Build history of the part. All positions in model axes, mm. A direction names the side the tool comes from. Coordinates: 2 decimals unless noted, no trailing zeros. Order: outer loops, then holes, each group sorted by start corner. A loop starts at its lowest first (then second) coordinate and runs counter-clockwise, first axis right, second up. Notation, with made-up numbers: (35, -18.5) - (77, -18.5) arc R18 ccw to (77, 12.5) - close; hole circle Ø4 at (-17, 80.25). An arc over 180 degrees is marked (long way). One line per item, written item: value.
Autodesk Inventor part; units mm, degrees
ref_plane "YZ Plane" through (0, 0, 0) normal (1, 0, 0) x (0, 1, 0)
ref_plane "XZ Plane" through (0, 0, 0) normal (0, 1, 0) x (-1, 0, 0)
ref_plane "XY Plane" through (0, 0, 0) normal (0, 0, 1) x (1, 0, 0)
sketch "草圖1" plane through (0, 0, 0) normal (0, 0, 1) x (1, 0, 0)
  circle A0 centre (0, 0) radius 20
  line L0 (0, -20) -> (0, -30)
  line L1 (0, -30) -> (70, -30)
  line L2 (70, -30) -> (70, -20)
  line L3 (70, -20) -> (40, 20)
  line L4 (40, 20) -> (0, 20)
  dimension "d0" = 40
  dimension "d1" = 10
  dimension "d2" = 70
  dimension "d3" = 40
  dimension "d4" = 10
extrude "擠出1" add sketch "草圖1" along normal blind 10
sketch "草圖2" plane through (0, 0, 10) normal (0, 0, 1) x (1, 0, 0)
  arc A0 (0, 20) -> (0, -20) centre (0, 0) ccw
hole "孔1" at (0, 0, 10) direction (0, 0, -1) diameter 20 end through all
sketch "草圖3" plane through (0, -30, 0) normal (0, -1, 0) x (1, 0, 0)
  line L0 (70, 10) -> (70, 0)
  line L1 (70, 0) -> (0, 0)
  line L2 (0, 0) -> (0, 10)
  line L3 (0, 10) -> (70, 10)
  circle A0 centre (20, 30) radius 20
  line L4 (0, 30) -> (40, 30)
  line L5 (40, 30) -> (40, 0)
  line L6 (40, 0) -> (0, 0)
  line L7 (0, 0) -> (0, 30)
  line L8 (0, 0) -> (70, 0)
  line L9 (0, 0) -> (0, 10)
  point P0 (40, 10)
  point P1 (40, 30)
  dimension "d14" = 40
  dimension "d15" = 30
extrude "擠出2" add sketch "草圖3" against normal blind 10 contours L3 A0 L5 | L3 L7 A0 | A0 L4 | L4 A0
sketch "草圖4" plane through (0, -20, 0) normal (0, 1, 0) x (1, 0, 0)
  arc A0 (0, -30) -> (40, -30) centre (20, -30) ccw
  point P0 (0, 0)
hole "孔2" at (20, -20, 30) direction (0, -1, 0) diameter 20 end through all
properties part number "25" material "鋼、碳鋼"
1. 3-axis set-ups, long thin cutter, end or side, ignore diameter. For faces 1 (the face through (40, -25, 20)), 2 (the face through (20, -20, 17)), 3 (the face through (55, 0, 5)): which of +Z, -Z, +X, -X, +Y, -Y reach the whole face in a straight line?
Values found:
face 1: +Z, +X, +Y, -Y
face 2: +Z, +X, -X, +Y
face 3: +Z, -Z, +X, +Y
2. Two-plate mould, pull along X, no slides. Class faces 4 (the face through (17, -25.07, 39.54)), 5 (the face through (20, 20, 5)), 6 (the face through (0, -25, 15)): pulls with the +X half, pulls with the -X half, needs draft (parallel to the pull), parting line crosses it, or undercut.
Values found:
face 4: undercut
face 5: needs draft
face 6: pulls with the -X half
3. Band-saw the part on A-A, the plane y = 0. Give the cut face in (x, z).
Values found:
outline: (-20, 0) - (-10, 0) - (-10, 10) - (-20, 10) - close; (10, 0) - (55, 0) - (55, 10) - (10, 10) - close
4. Band-saw the part on B-B, the plane x = 20. Give the cut face in (y, z).
Values found:
outline: (-30, 0) - (20, 0) - (20, 10) - (-20, 10) - (-20, 20) - (-30, 20) - close; (-30, 40) - (-20, 40) - (-20, 50) - (-30, 50) - close
5. Flat gauge pins, fed straight in: P1, Ø3, axis at y = -21, z = 23.5, coming from the +X side; P2, Ø12, axis at x = 14.5, z = 30, coming from the +Y side; P3, Ø11, axis at y = -25.5, z = 22.5, coming from the -X side. Where does each tip first touch, or does it go through?
Values found:
P1: stops at x = 40
P2: stops at y = -20
P3: stops at x = 0
6. Band-saw the part on C-C, the plane z = 32. Give the cut face in (x, y).
Values found:
outline: (0.1, -30) - (10.2, -30) - (10.2, -20) - (0.1, -20) - close; (29.8, -30) - (39.9, -30) - (39.9, -20) - (29.8, -20) - close
7. Band-saw the part on D-D, the plane z = 11. Give the cut face in (x, y).
Values found:
outline: (0, -30) - (40, -30) - (40, -20) - (0, -20) - close
8. Probe line 1 along X through (y, z) = (-25, 30); line 2 along Z through (x, y) = (18, -10); line 3 along Y through (x, z) = (4, 21.5). List the from-to ranges inside material, lowest first.
Values found:
line 1: x = 0 to 10, 30 to 40
line 2: z = 0 to 10
line 3: y = -30 to -20
